Check sheet for the modelled part. Datum: model origin and axes. Units: mm. A direction names the side the tool comes from. Round coordinates to 2 decimals unless told otherwise and drop trailing zeros. Write each loop counter-clockwise with the first axis right and the second up, starting at its lowest first coordinate (ties: lowest second). Pieces come first, ordered by that corner, then holes. Notation, with made-up numbers: (45.5, 46) - (99.5, 46) arc R13 cw to (99.5, 52) - close; hole circle Ø8 at (-39.5, 65). An arc over 180 degrees is marked (long way). Use one line per item in the form item = value. Start each with the question number.
1) Section check A-A (y = 7.73). Record the boundary of the cut face in (x, z), then the cut area to 3 significant figures.
2) Set-up check for faces 1 (the face through (10, -9, -8)), 2 (the face through (0, 3.5, 2)), 3 (the face through (21, -4, -2)), 4 (the face through (26.83, -7.01, -3.25)): record each of +Z, -Z, +X, -X, +Y, -Y from which the full face is reachable in a straight line by a thin tool's end or side.
3) Section check C-C (x = 28.5). Record the boundary of the cut face in (y, z), then the cut area to 3 significant figures.
4) Gauge pin test, flat ends, axial feed: P1, Ø2, axis at y = -3.5, z = 33.5, coming from the +X side; P2, Ø5.5, axis at y = -3.5, z = 40.5, coming from the -X side; P3, Ø1.2, axis at x = 7, z = 1.5, coming from the +Y side; P4, Ø2, axis at x = -19.5, y = 32, coming from the -Z side. Record the tip position at first contact, or that the pin passes through.
5) Draft check along Z on faces 5 (the face through (-26.83, 36.284, -5.07)), 6 (the face through (-26.83, 41.354, -5.422)), 7 (the face through (-27, 40.27, 2)), 8 (the face through (23.898, -3.303, 29.276)). Enter one of: +Z half, -Z half, draft (parallel to the pull), parting line (faces both ways), or undercut.
6) Section check B-B (z = 19). Record the boundary of the cut face in (x, y).
7) Section check D-D (z = -4.5). Record the boundary of the cut face in (x, y), then the cut area to 3 significant figures.
8) Scan lines: probe 1 along Y at (x, z) = (-28.5, 2.65); probe 2 along Y at (x, z) = (28, 1); probe 3 along X at (y, z) = (-45.25, -7.35). Record each from-to range of solid material in increasing order.
from build123d import *

# Parameters (mm, degrees)
SKETCH1_R            = 1.7
BOSS_EXTRUDE1_DEPTH  = 4
BOSS_EXTRUDE7_DEPTH  = 65
SKETCH9_W            = 42
SKETCH9_H            = 10.1
CUT_EXTRUDE2_DEPTH   = 2
SKETCH4_W            = 65
SKETCH4_H            = 3.9
BOSS_EXTRUDE3_DEPTH  = 52
SKETCH5_R            = 1.6
CUT_EXTRUDE1_DEPTH   = 50
BOSS_EXTRUDE8_START  = -10
BOSS_EXTRUDE8_DEPTH  = 32.27
FILLET1_R            = 10
BOSS_EXTRUDE9_DEPTH  = 11.5
BOSS_EXTRUDE12_START = -65
BOSS_EXTRUDE12_DEPTH = 11.5
FILLET5_R            = 10
SKETCH14_W           = 12
SKETCH14_H           = 15
SKETCH14_W_2         = 11.826086957
BOSS_EXTRUDE10_DEPTH = 5
FILLET3_R            = 10
SKETCH15_W           = 22
SKETCH15_H           = 30
CUT_EXTRUDE3_DEPTH   = 10
FILLET6_R            = 5
FILLET7_R            = 10
BOSS_EXTRUDE13_REACH = 95.361
FILLET8_R            = 10
FILLET9_R            = 5
FILLET10_START       = -2
FILLET10_DEPTH       = 32.27
FILLET10_START_2     = -32.5
FILLET10_2_DEPTH     = 65
FILLET10_START_3     = 20.99999979
FILLET10_3_DEPTH     = 4.00000021
FILLET10_START_4     = -25
FILLET10_4_DEPTH     = 4
FILLET10_START_5     = 30.27
FILLET10_5_DEPTH     = 12.000012257


with BuildPart() as part:
    # Sketch1 → Boss-Extrude1 (new body)
    with BuildSketch(Plane.XY):
        Polygon((-21, 40.27), (-21, 3.5), (21, 3.5), (21, 40.27), (32.5, 40.27), (32.5, 0), (-32.5, 0), (-32.5, 40.27), align=None)
        with Locations((-28.5, 27.73)):
            Circle(SKETCH1_R, mode=Mode.SUBTRACT)
        with Locations((-28.5, 7.73)):
            Circle(SKETCH1_R, mode=Mode.SUBTRACT)
        with Locations(Location((28.5, 7.73, 0), (0, 0, 180))):
            Circle(SKETCH1_R, mode=Mode.SUBTRACT)
        with Locations(Location((28.5, 27.73, 0), (0, 0, 180))):
            Circle(SKETCH1_R, mode=Mode.SUBTRACT)
    extrude(amount=BOSS_EXTRUDE1_DEPTH)

    # Sketch7 → Boss-Extrude7 (add)
    with BuildSketch(Plane(origin=(32.5, 0, 0), x_dir=(0, 0, -1), z_dir=(1, 0, 0))):
        Polygon((0, 0), (-4, 0), (-4, -4), (10, -4), (10, 0.674077793), (0, 0.15), align=None)
    extrude(amount=-BOSS_EXTRUDE7_DEPTH)

    # Sketch9 → Cut-Extrude2 (cut)
    with BuildSketch(Plane.XZ.offset(4)):
        with Locations((0, -1.05)):
            Rectangle(SKETCH9_W, SKETCH9_H)
    extrude(amount=-CUT_EXTRUDE2_DEPTH, mode=Mode.SUBTRACT)

    # Sketch4 → Boss-Extrude3 (add)
    with BuildSketch(Plane.XZ.offset(4)):
        with Locations((0, -8.05)):
            Rectangle(SKETCH4_W, SKETCH4_H)
    extrude(amount=BOSS_EXTRUDE3_DEPTH)

    # Sketch5 → Cut-Extrude1 (cut)
    with BuildSketch(Plane.XY.offset(-10)):
        with Locations(Location((-15.5, -45.25, 0), (0, 0, 180))):
            Circle(SKETCH5_R)
        with Locations(Location((15.5, -45.25, 0), (0, 0, 180))):
            Circle(SKETCH5_R)
    extrude(amount=CUT_EXTRUDE1_DEPTH, mode=Mode.SUBTRACT)

    # Sketch11 → Boss-Extrude8 (add)
    with BuildSketch(Plane(origin=(0, 40.27, 0), x_dir=(1, 0, 0), z_dir=(0, 1, 0)).offset(BOSS_EXTRUDE8_START)):
        Polygon((-23, -4), (-25, -4), (-25, -50), (25, -50), (25, -4), (22.826086957, -4), (22.826086957, -48), (-23, -48), align=None)
    extrude(amount=-BOSS_EXTRUDE8_DEPTH)

    # Fillet1
    fillet1_edges = [part.edges().sort_by_distance(p)[0] for p in [
        (-26.75, -4, -6.1),
        (26.75, -4, -6.1),
    ]]
    fillet(fillet1_edges, radius=FILLET1_R)

    # Sketch13 → Boss-Extrude9 (add)
    with BuildSketch(Plane(origin=(32.5, 0, 0), x_dir=(0, 0, -1), z_dir=(1, 0, 0))):
        Polygon((10, 42.270012257), (0, 40.27), (0, 35.27), (10, 37.270012257), align=None)
    extrude(amount=-BOSS_EXTRUDE9_DEPTH)

    # Sketch13<8> → Boss-Extrude12 (add)
    with BuildSketch(Plane(origin=(32.5, 0, 0), x_dir=(0, 0, -1), z_dir=(1, 0, 0)).offset(BOSS_EXTRUDE12_START)):
        Polygon((0, 40.27), (10, 42.270012257), (10, 37.270012257), (0, 35.27), align=None)
    extrude(amount=BOSS_EXTRUDE12_DEPTH)

    # Fillet5
    fillet5_edges = [part.edges().sort_by_distance(p)[0] for p in [
        (-26.75, 40.27, 0),
        (26.75, 40.27, 0),
    ]]
    fillet(fillet5_edges, radius=FILLET5_R)

    # Sketch14 → Boss-Extrude10 (add)
    with BuildSketch(Plane.XZ.offset(2)):
        with Locations((-17, 40.5)):
            Rectangle(SKETCH14_W, SKETCH14_H)
        with Locations((16.913043479, 40.5)):
            Rectangle(SKETCH14_W_2, SKETCH14_H)
        Polygon((25, 50), (11, 50), (11, 48), (22.826086957, 48), (22.826086957, 33), (25, 33), align=None)
        Polygon((-11, 50), (-25, 50), (-25, 33), (-23, 33), (-23, 48), (-11, 48), align=None)
    extrude(amount=BOSS_EXTRUDE10_DEPTH)

    # Fillet3
    # the kernel refuses this fillet: 10 mm, written as the material it adds along each edge
    with BuildSketch(Plane(origin=(22.826086957, -2, 33), x_dir=(0, -1, 0), z_dir=(1, 0, 0))) as fillet3_piece_1:
        with BuildLine():
            CenterArc((10, 8.660254038), FILLET3_R, 180, 60)
            Line((0, 8.660254038), (0, 0))
            Line((0, 0), (5, 0))
        make_face()
    extrude(amount=2.173913043)
    with BuildSketch(Plane(origin=(-25, -2, 33), x_dir=(0, -1, 0), z_dir=(1, 0, 0)), Plane(origin=(11, -2, 50), x_dir=(0, -1, 0), z_dir=(0, 0, -1))) as fillet3_piece_2:
        with BuildLine():
            CenterArc((10, 8.660254038), FILLET3_R, 180, 60)
            Line((0, 8.660254038), (0, 0))
            Line((0, 0), (5, 0))
        make_face()
    extrude(amount=2)
    with BuildSketch(Plane(origin=(-11, -2, 48), x_dir=(1, 0, 0), z_dir=(0, 0, 1))) as fillet3_piece_3:
        with BuildLine():
            CenterArc((8.660254038, -10), FILLET3_R, 90, 60)
            Line((0, -5), (0, 0))
            Line((0, 0), (8.660254038, 0))
        make_face()
    extrude(amount=2)

    # Sketch15 → Cut-Extrude3 (cut)
    with BuildSketch(Plane.XY.offset(-6.1)):
        with Locations((0, -22)):
            Rectangle(SKETCH15_W, SKETCH15_H)
        Polygon((-32.5, -14), (-20, -56), (-32.5, -56), align=None)
        Polygon((32.5, -56), (20, -56), (32.5, -14), align=None)
    extrude(amount=-CUT_EXTRUDE3_DEPTH, mode=Mode.SUBTRACT)

    # Fillet6
    fillet6_edges = [part.edges().sort_by_distance(p)[0] for p in [
        (-11, -37, -8.05),
        (-11, -7, -8.05),
        (11, -7, -8.05),
        (11, -37, -8.05),
    ]]
    fillet(fillet6_edges, radius=FILLET6_R)

    # Fillet7
    fillet7_edges = [part.edges().sort_by_distance(p)[0] for p in [
        (-20, -56, -8.05),
        (-32.5, -14, -8.05),
        (32.5, -14, -8.05),
        (20, -56, -8.05),
    ]]
    fillet(fillet7_edges, radius=FILLET7_R)

    # Boss-Extrude13: up to this face of the body (flat: up to its plane)
    boss_extrude13_end = Plane(part.part.faces().sort_by_distance((22.826086957, 13.980833311, 26.043580166))[0])
    # Sketch16 → Boss-Extrude13 (add, up to the picked face)
    with BuildSketch(Plane(origin=(-23, 0, 0), x_dir=(0, 0, -1), z_dir=(1, 0, 0)), mode=Mode.PRIVATE) as boss_extrude13_sk1:
        Polygon((-4, -2), (-4, 3.5), (-13.5, -2), align=None)
    boss_extrude13_tool1 = split(extrude(boss_extrude13_sk1.sketch, amount=BOSS_EXTRUDE13_REACH, mode=Mode.PRIVATE), bisect_by=boss_extrude13_end, keep=Keep.BOTH, mode=Mode.PRIVATE)
    add(boss_extrude13_tool1.solids().sort_by(Axis((-23, -0.166667, 7.166667), (1, 0, 0)))[0])

    # Fillet8
    # the kernel refuses this fillet: 10 mm, written as the material it adds along each edge
    with BuildSketch(Plane(origin=(-21, -2, 4), x_dir=(0, -1, 0), z_dir=(-1, 0, 0)), Plane(origin=(25, -2, 4), x_dir=(0, -1, 0), z_dir=(-1, 0, 0))) as fillet8_piece_1:
        with BuildLine():
            CenterArc((10, 6), FILLET8_R, 180, 36.869897646)
            Line((0, 6), (-0.2, 6))
            Line((-0.2, 6), (-0.2, 0))
            Line((-0.2, 0), (0, -0.2))
            ThreePointArc((0, -0.2), (1, -0.2), (1.84, -0.12))
            Line((1.84, -0.12), (2, 0))
        make_face()
    extrude(amount=4)

    # Fillet9
    # the kernel refuses this fillet: 5 mm, written as the material it adds along each edge
    with BuildSketch(Plane(origin=(22.826086957, 30.27, 4), x_dir=(-1, 0, 0), z_dir=(0, -1, 0))) as fillet9_piece_1_section:
        with BuildLine():
            CenterArc((5, -3.863453894), FILLET9_R, 129.403862825, 50.596137175)
            Line((0, -3.863453894), (0, 0))
            Line((0, 0), (1.826086957, 0))
        make_face()
    fillet9_piece_1 = extrude(amount=36.428634735, mode=Mode.PRIVATE)
    fillet9_piece_1 = split(fillet9_piece_1, bisect_by=Plane(origin=(22.826086957, -2, 4), z_dir=(0, 1, 0)), keep=Keep.TOP, mode=Mode.PRIVATE)
    add(fillet9_piece_1)
    with BuildSketch(Plane(origin=(-23, 30.27, 4), x_dir=(0, 0, 1), z_dir=(0, -1, 0))) as fillet9_piece_2_section:
        with BuildLine():
            CenterArc((4, -5), FILLET9_R, 90, 53.130102354)
            Line((0, -2), (0, 0))
            Line((0, 0), (4, 0))
        make_face()
    fillet9_piece_2 = extrude(amount=36.77, mode=Mode.PRIVATE)
    fillet9_piece_2 = split(fillet9_piece_2, bisect_by=Plane(origin=(-23, -2, 4), z_dir=(0, 1, 0)), keep=Keep.TOP, mode=Mode.PRIVATE)
    add(fillet9_piece_2)

    # Fillet10: read off the stored shape, not the designer's step
    # Fillet10 outline → Fillet10 (add)
    with BuildSketch(Plane(origin=(0, 0, 0), x_dir=(1, 0, 0), z_dir=(0, 1, 0)).offset(FILLET10_START)):
        with BuildLine():
            Line((-23, -48), (-13, -48))
            ThreePointArc((-13, -48), (-20.071067812, -45.071067812), (-23, -38))
            Line((-23, -38), (-23, -48))
        make_face()
        with BuildLine():
            ThreePointArc((22.826086957, -38), (19.897154769, -45.071067812), (12.826086957, -48))
            Line((12.826086957, -48), (22.826086957, -48))
            Line((22.826086957, -48), (22.826086957, -38))
        make_face()
    extrude(amount=FILLET10_DEPTH)

    # Fillet10 2 outline → Fillet10 2 (cut)
    with BuildSketch(Plane.YZ.offset(FILLET10_START_2)):
        with BuildLine():
            ThreePointArc((-7, 40), (-4.071067812, 47.071067812), (3, 50))
            Line((3, 50), (-7, 50))
            Line((-7, 50), (-7, 40))
        make_face()
    extrude(amount=FILLET10_2_DEPTH, mode=Mode.SUBTRACT)

    # Fillet10 3 outline → Fillet10 3 (add)
    with BuildSketch(Plane.YZ.offset(FILLET10_START_3)):
        with BuildLine():
            ThreePointArc((40.27, 4), (33.198932188, 6.928932188), (30.27, 14))
            Line((30.27, 14), (30.27, 4))
            Line((30.27, 4), (40.27, 4))
        make_face()
    extrude(amount=FILLET10_3_DEPTH)

    # Fillet10 4 outline → Fillet10 4 (add)
    with BuildSketch(Plane.YZ.offset(FILLET10_START_4)):
        with BuildLine():
            ThreePointArc((40.27, 4), (33.198932188, 6.928932188), (30.27, 14))
            Line((30.27, 14), (30.27, 4))
            Line((30.27, 4), (40.27, 4))
        make_face()
    extrude(amount=FILLET10_4_DEPTH)

    # Fillet10 5 outline → Fillet10 5 (cut)
    with BuildSketch(Plane(origin=(0, 0, 0), x_dir=(1, 0, 0), z_dir=(0, 1, 0)).offset(FILLET10_START_5)):
        with BuildLine():
            ThreePointArc((22.826086957, -7.863453894), (22.346570275, -5.726813876), (20.999994729, -3.99999567))
            Line((20.999994729, -3.99999567), (20.99999979, -14))
            Line((20.99999979, -14), (20.99999979, -15))
            Line((20.99999979, -15), (22.826086959, -15))
            Line((22.826086959, -15), (22.826086957, -7.863453894))
        make_face()
        with BuildLine():
            Line((-22.999999999, -15), (-21, -15))
            Line((-21, -15), (-21, -14))
            Line((-21, -14), (-20.9999923, -3.999994225))
            ThreePointArc((-20.9999923, -3.999994225), (-22.472133803, -5.763927718), (-23, -8))
            Line((-23, -8), (-22.999999999, -15))
        make_face()
    extrude(amount=FILLET10_5_DEPTH, mode=Mode.SUBTRACT)


solid = part.part
Results are:
q1.outline = (-32.5, 0) - (-30.2, 0) - (-30.2, 4) - (-32.5, 4) - close; (-26.8, 0) - (-21, 0) - (-21, 4) arc R5 cw to (-23, 8) - (-23, 38) arc R10 cw to (-13, 48) - (12.83, 48) arc R10 cw to (22.83, 38) - (22.83, 7.86) arc R5 cw to (21, 4) - (21, 0) - (26.8, 0) - (26.8, 4) - (25, 4) - (25, 50) - (-25, 50) - (-25, 4) - (-26.8, 4) - close; (30.2, 0) - (32.5, 0) - (32.5, 4) - (30.2, 4) - close
q1.area = 396 mm²
q2.face_1 = +Z, -Z
q2.face_2 = -Z, +Y
q2.face_3 = -Y
q2.face_4 = +X, -X, -Y
q3.outline = (-27.44, -10) - (0.67, -10) - (0.15, 0) - (6.03, 0) - (6.03, 4) - (-4, 4) - (-4, 3.9) arc R10 cw to (-14, -6.1) - (-27.44, -6.1) - close; (9.43, 0) - (26.03, 0) - (26.03, 4) - (9.43, 4) - close; (29.43, 0) - (35.27, 0) - (37.27, -10) - (42.27, -10) - (40.46, -0.97) arc R10 cw to (40.27, 0.99) - (40.27, 4) - (29.43, 4) - close
q3.area = 357 mm²
q4.P1 = 25
q4.P2 = -25
q4.P3 = 3.5
q4.P4 = through
q5.face_5 = -Z half
q5.face_6 = +Z half
q5.face_7 = draft
q5.face_8 = undercut
q6.outline = (-25, -2) - (-23, -2) - (-23, 30.27) - (-25, 30.27) - close; (22.83, -2) - (25, -2) - (25, 30.27) - (22.83, 30.27) - close
q7.outline = (-32.5, -8.57) - (-21, -8.57) - (-21, -2) - (21, -2) - (21, -8.57) - (32.5, -8.57) - (32.5, 0.39) - (-32.5, 0.39) - close; (-32.5, 36.17) - (-21, 36.17) - (-21, 41.17) - (-32.5, 41.17) - close; (21, 36.17) - (32.5, 36.17) - (32.5, 41.17) - (21, 41.17) - close
q7.area = 421 mm²
q8.probe_1 = -4.08 to 6.03, 9.43 to 26.03, 29.43 to 40.27
q8.probe_2 = -4.43 to 6.11, 9.35 to 26.11, 29.35 to 40.27
q8.probe_3 = -23.2 to -17.1, -13.9 to 13.9, 17.1 to 23.2
